Part model, mm, in its own coordinate system. Coordinates: 2 decimals unless noted, no trailing zeros. Loops run counter-clockwise (first coordinate to the right, second up) from the corner with the lowest first, then second, coordinate; pieces in that order, holes last. Notation, with made-up numbers: (-40, 6) - (-35, 6) arc R12 cw to (-35, 25) - close; hole circle Ø7 at (-2.75, 33). An arc over 180 degrees is marked (long way). Answer as CSV lines item,"result".
from build123d import *

# Parameters (mm, degrees)
BOSS_EXTRUDE1_DEPTH = 0.5
SKETCH2_W           = 21
SKETCH2_H           = 19.8
BOSS_EXTRUDE2_DEPTH = 0.5
SKETCH3_W           = 13
SKETCH3_H           = 0.5
CUT_EXTRUDE1_DEPTH  = 25.442919676


with BuildPart() as part:
    # Sketch1 → Boss-Extrude1 (new body)
    with BuildSketch(Plane(origin=(0, 0, 0), x_dir=(1, 0, 0), z_dir=(0, 1, 0))):
        Polygon((-15.118410045, 7.342838361), (-15.118410045, -12.457161639), (-14.518410045, -12.457161639), (-14.518410045, 6.742838361), (5.281589955, 6.742838361), (5.281589955, -12.457161639), (5.881589955, -12.457161639), (5.881589955, 7.342838361), align=None)
    extrude(amount=BOSS_EXTRUDE1_DEPTH)

    # Sketch2 → Boss-Extrude2 (add)
    with BuildSketch(Plane.XZ):
        with Locations((-4.618410045, 2.557161639)):
            Rectangle(SKETCH2_W, SKETCH2_H)
    extrude(amount=BOSS_EXTRUDE2_DEPTH)

    # Sketch3 → Cut-Extrude1 (cut, through all)
    with BuildSketch(Plane.XY.offset(-6.742838361)):
        with Locations((-4.618410045, 0.25)):
            Rectangle(SKETCH3_W, SKETCH3_H)
    extrude(amount=-CUT_EXTRUDE1_DEPTH, mode=Mode.SUBTRACT)


solid = part.part
Q1. Saw through at A-A (y = 0.35). Give the cut face in (x, z), then the cut area to 3 significant figures.
Results:
outline,"(-15.12, -7.34) - (-11.12, -7.34) - (-11.12, -6.74) - (-14.52, -6.74) - (-14.52, 12.46) - (-15.12, 12.46) - close; (1.88, -7.34) - (5.88, -7.34) - (5.88, 12.46) - (5.28, 12.46) - (5.28, -6.74) - (1.88, -6.74) - close"
area,"27.8 mm^2"
Q2. Wall check: L1, parallel to X at y = 0.25, z = 10.75; L2, parallel to Y at x = -7.5, z = 3.5; L3, parallel to Z at x = -12.75, y = 0.3. Give the ranges that are in metal, low to high.
Results:
L1,"x = -15.12 to -14.52, 5.28 to 5.88"
L2,"y = -0.5 to 0"
L3,"z = -7.34 to -6.74"
Q3. Saw through at B-B (z = 9.75). Give the cut face in (x, y), then the cut area to 3 significant figures.
Results:
outline,"(-15.12, -0.5) - (5.88, -0.5) - (5.88, 0.5) - (5.28, 0.5) - (5.28, 0) - (-14.52, 0) - (-14.52, 0.5) - (-15.12, 0.5) - close"
area,"11.1 mm^2"
Q4. Flat gauge pins, fed straight in: pin 1 (5 mm diameter, centred on x = 2.5, z = 3, fed in from +Y); pin 2 (0.6 mm diameter, centred on x = 3.5, y = 0.5, fed in from +Z). Where does each tip first touch, or does it go through?
Results:
pin 1,"stops at y = 0"
pin 2,"stops at z = -6.74"
Q5. Saw through at D-D (x = -0.5). Give the cut face in (y, z).
Results:
outline,"(-0.5, -7.34) - (0, -7.34) - (0, 12.46) - (-0.5, 12.46) - close"
Q6. Saw through at C-C (x = -12.5). Give the cut face in (y, z), then the cut area to 3 significant figures.
Results:
outline,"(-0.5, -7.34) - (0.5, -7.34) - (0.5, -6.74) - (0, -6.74) - (0, 12.46) - (-0.5, 12.46) - close"
area,"10.2 mm^2"
